Here's how the part is built. I have some questions about the finished solid (model axes, mm). A direction names the side the tool comes from. Round coordinates to 2 decimals unless told otherwise and drop trailing zeros. Order: outer loops, then holes, each group sorted by start corner. A loop starts at its lowest first (then second) coordinate and runs counter-clockwise, first axis right, second up.
```python
from build123d import *

# Parameters (mm, degrees)
BOSS_EXTRUDE1_DEPTH = 3
SKETCH2_R           = 1.75
CUT_EXTRUDE1_DEPTH  = 65.356450115


with BuildPart() as part:
    # Sketch1 → Boss-Extrude1 (new body)
    with BuildSketch(Plane(origin=(0, 0, 0), x_dir=(1, 0, 0), z_dir=(0, 1, 0))):
        Polygon((-41.611393926, 23.081435644), (41.611393926, 23.081435644), (60, -8.768564356), (60, -17.418564356), (38.5, -17.418564356), (38.5, 20.081435644), (-38.5, 20.081435644), (-38.5, -17.418564356), (-60, -17.418564356), (-60, -8.768564356), align=None)
    extrude(amount=BOSS_EXTRUDE1_DEPTH)

    # Sketch2 → Cut-Extrude1 (cut, through all)
    with BuildSketch(Plane(origin=(0, 3, 0), x_dir=(1, 0, 0), z_dir=(0, 1, 0))):
        with Locations(Location((52, -9.918564356, 0), (0, 0, 270))):
            Circle(SKETCH2_R)
        with Locations(Location((44, -9.918564356, 0), (0, 0, 270))):
            Circle(SKETCH2_R)
        with Locations(Location((-52, -9.918564356, 0), (0, 0, 90))):
            Circle(SKETCH2_R)
        with Locations(Location((-44, -9.918564356, 0), (0, 0, 90))):
            Circle(SKETCH2_R)
    extrude(amount=-CUT_EXTRUDE1_DEPTH, mode=Mode.SUBTRACT)


solid = part.part
```
1. If we section it at A-A, the plane x = -44: Write out the boundary of the cut face in (y, z), and give its area (3 significant figures).
Evaluation:
outline: (0, -18.94) - (3, -18.94) - (3, 8.17) - (0, 8.17) - close; (0, 11.67) - (3, 11.67) - (3, 17.42) - (0, 17.42) - close
area: 98.6 mm2
2. If we section it at B-B, the plane z = 5.5: Write out the boundary of the cut face in (x, y).
Evaluation:
outline: (-58.11, 0) - (-38.5, 0) - (-38.5, 3) - (-58.11, 3) - close; (38.5, 0) - (58.11, 0) - (58.11, 3) - (38.5, 3) - close
3. I'm going to push flat-ended pins straight in: P1, Ø1.5, axis at x = -7, y = 0.5, coming from the +Z side; P2, Ø12, axis at x = 36, z = -15.5, coming from the -Y side; P3, Ø0.9, axis at y = 1.5, z = -10.5, coming from the -X side; P4, Ø1.5, axis at y = 2, z = 2.5, coming from the +X side. Where does each tip first touch, or does it pass through?
Evaluation:
P1: stops at z = -20.08
P2: stops at y = 0
P3: stops at x = -49.14
P4: stops at x = 56.81
4. If we section it at D-D, the plane z = 10: Write out the boundary of the cut face in (x, y).
Evaluation:
outline: (-60, 0) - (-53.75, 0) - (-53.75, 3) - (-60, 3) - close; (-50.25, 0) - (-45.75, 0) - (-45.75, 3) - (-50.25, 3) - close; (-42.25, 0) - (-38.5, 0) - (-38.5, 3) - (-42.25, 3) - close; (38.5, 0) - (42.25, 0) - (42.25, 3) - (38.5, 3) - close; (45.75, 0) - (50.25, 0) - (50.25, 3) - (45.75, 3) - close; (53.75, 0) - (60, 0) - (60, 3) - (53.75, 3) - close
5. I need wall thicknesses on probe 1 along X at (y, z) = (1.9, 11.5); probe 2 along Z at (x, y) = (-10, 1.35); probe 3 along X at (y, z) = (0.2, -3). Which ranges of each line are inside material? Lowest first, please.
Evaluation:
probe 1: x = -60 to -52.75, -51.25 to -44.75, -43.25 to -38.5, 38.5 to 43.25, 44.75 to 51.25, 52.75 to 60
probe 2: z = -23.08 to -20.08
probe 3: x = -53.21 to -38.5, 38.5 to 53.21
6. If we section it at C-C, the plane y = 2.5: Write out the boundary of the cut face in (x, z), and give its area (3 significant figures).
Evaluation:
outline: (-60, 8.77) - (-41.61, -23.08) - (41.61, -23.08) - (60, 8.77) - (60, 17.42) - (38.5, 17.42) - (38.5, -20.08) - (-38.5, -20.08) - (-38.5, 17.42) - (-60, 17.42) - close; hole circle Ø3.5 at (-52, 9.92); hole circle Ø3.5 at (-44, 9.92); hole circle Ø3.5 at (44, 9.92); hole circle Ø3.5 at (52, 9.92)
area: 1,350 mm2
7. On a 3-axis mill with a long thin cutter (end or side, diameter ignored), from which of +Z, -Z, +X, -X, +Y, -Y can I reach the whole of each face in a straight line? I mean faces 4 (the flat face through (-38.5, 1, -2)), 5 (the flat face through (49, 1, 17.419)). Say none if no direction works.
Evaluation:
face 4: +Z, +Y, -Y
face 5: +Z, +X, -X, +Y, -Y
8. If we mould it in two halves opening along X, with no side actions, what happens to faces 1 (the flat face through (-49, 1, 17.419)), 2 (the cylindrical face through (-42.292, 1.521, 10.298)), 3 (the flat face through (-50.934, 1.479, -6.933))? For each: released by +X, released by -X, zero draft, split by the parting line, or undercut.
Evaluation:
face 1: zero draft
face 2: undercut
face 3: released by -X
